For this review, take the finished solid that the model builds, in its own axes (mm). A direction names the side the tool comes from. Give positions to 0.01 mm unless a question says otherwise; leave off trailing zeros. Loops run counter-clockwise (first coordinate to the right, second up) from the corner with the lowest first, then second, coordinate; pieces in that order, holes last. Notation, with made-up numbers: (-1.75, 18) - (23.25, 18) arc R23 ccw to (23.25, 47) - close; hole circle Ø9 at (66, -6.75). An arc over 180 degrees is marked (long way). Put each result on its own line as item: value.
from build123d import *

# Parameters (mm, degrees)
CUT_EXTRUDE1_START = -1828.8
CUT_EXTRUDE1_DEPTH = 660.4
SKETCH3_R          = 2.38125
CUT_EXTRUDE3_DEPTH = 50.8
CUT_EXTRUDE4_REACH = 664.838
SKETCH4_R          = 2.413
CUT_EXTRUDE5_REACH = 664.838
SKETCH5_R          = 2.85115
SKETCH6_R          = 2.38125
CUT_EXTRUDE6_DEPTH = 663.837808315


with BuildPart() as part:
    # Cut-Extrude1: read off the stored shape, not the designer's step
    # Cut-Extrude1 outline → Cut-Extrude1 (new body)
    with BuildSketch(Plane.XY.offset(1828.8).offset(CUT_EXTRUDE1_START)):
        with BuildLine():
            Line((0, 50.546), (0, 0.254))
            ThreePointArc((0, 0.254), (0.074394878, 0.074394878), (0.254, 0))
            Line((0.254, 0), (25.146, 0))
            ThreePointArc((25.146, 0), (25.325605122, 0.074394878), (25.4, 0.254))
            Line((25.4, 0.254), (25.4, 50.546))
            ThreePointArc((25.4, 50.546), (25.325605122, 50.725605122), (25.146, 50.8))
            Line((25.146, 50.8), (0.254, 50.8))
            ThreePointArc((0.254, 50.8), (0.074394878, 50.725605122), (0, 50.546))
        make_face()
        with BuildLine():
            ThreePointArc((4.7625, 3.175), (3.639967985, 3.639967985), (3.175, 4.7625))
            Line((3.175, 4.7625), (3.175, 46.0375))
            ThreePointArc((3.175, 46.0375), (3.639967985, 47.160032015), (4.7625, 47.625))
            Line((4.7625, 47.625), (20.6375, 47.625))
            ThreePointArc((20.6375, 47.625), (21.760032015, 47.160032015), (22.225, 46.0375))
            Line((22.225, 46.0375), (22.225, 4.7625))
            ThreePointArc((22.225, 4.7625), (21.760032015, 3.639967985), (20.6375, 3.175))
            Line((20.6375, 3.175), (4.7625, 3.175))
        make_face(mode=Mode.SUBTRACT)
    extrude(amount=CUT_EXTRUDE1_DEPTH)

    # Sketch3 → Cut-Extrude3 (cut)
    with BuildSketch(Plane(origin=(0, 50.8, 0), x_dir=(1, 0, 0), z_dir=(0, 1, 0))):
        with Locations(Location((12.7, -25.4, 0), (0, 0, 270))):
            Circle(SKETCH3_R)
        with Locations(Location((12.7, -12.7, 0), (0, 0, 270))):
            Circle(SKETCH3_R)
        with Locations(Location((12.7, -38.1, 0), (0, 0, 270))):
            Circle(SKETCH3_R)
        with Locations(Location((12.7, -622.3, 0), (0, 0, 270))):
            Circle(SKETCH3_R)
        with Locations(Location((12.7, -635, 0), (0, 0, 270))):
            Circle(SKETCH3_R)
        with Locations(Location((12.7, -647.7, 0), (0, 0, 270))):
            Circle(SKETCH3_R)
    extrude(amount=-CUT_EXTRUDE3_DEPTH, mode=Mode.SUBTRACT)

    # Sketch4 → Cut-Extrude4 (cut, up to next)
    with BuildSketch(Plane(origin=(0, 50.8, 0), x_dir=(1, 0, 0), z_dir=(0, 1, 0)), mode=Mode.PRIVATE) as cut_extrude4_sk1:
        with Locations(Location((12.7, -532.289940881, 0), (0, 0, 270))):
            Circle(SKETCH4_R)
    cut_extrude4_tool1 = extrude(cut_extrude4_sk1.sketch, amount=-CUT_EXTRUDE4_REACH, mode=Mode.PRIVATE) & part.part
    # Sketch4 → Cut-Extrude4 (cut, up to next)
    with BuildSketch(Plane(origin=(0, 50.8, 0), x_dir=(1, 0, 0), z_dir=(0, 1, 0)), mode=Mode.PRIVATE) as cut_extrude4_sk2:
        with Locations(Location((12.7, -506.889940881, 0), (0, 0, 270))):
            Circle(SKETCH4_R)
    cut_extrude4_tool2 = extrude(cut_extrude4_sk2.sketch, amount=-CUT_EXTRUDE4_REACH, mode=Mode.PRIVATE) & part.part
    add(cut_extrude4_tool1.solids().sort_by_distance((12.7, 50.8, 532.289941))[0], mode=Mode.SUBTRACT)
    add(cut_extrude4_tool2.solids().sort_by_distance((12.7, 50.8, 506.889941))[0], mode=Mode.SUBTRACT)

    # Sketch5 → Cut-Extrude5 (cut, up to next)
    with BuildSketch(Plane(origin=(25.4, 0, 0), x_dir=(0, 0, -1), z_dir=(1, 0, 0)), mode=Mode.PRIVATE) as cut_extrude5_sk1:
        with Locations((-462.47685, 31.33725)):
            Circle(SKETCH5_R)
    cut_extrude5_tool1 = extrude(cut_extrude5_sk1.sketch, amount=-CUT_EXTRUDE5_REACH, mode=Mode.PRIVATE) & part.part
    # Sketch5 → Cut-Extrude5 (cut, up to next)
    with BuildSketch(Plane(origin=(25.4, 0, 0), x_dir=(0, 0, -1), z_dir=(1, 0, 0)), mode=Mode.PRIVATE) as cut_extrude5_sk2:
        with Locations((-429.82515, 31.33725)):
            Circle(SKETCH5_R)
    cut_extrude5_tool2 = extrude(cut_extrude5_sk2.sketch, amount=-CUT_EXTRUDE5_REACH, mode=Mode.PRIVATE) & part.part
    # Sketch5 → Cut-Extrude5 (cut, up to next)
    with BuildSketch(Plane(origin=(25.4, 0, 0), x_dir=(0, 0, -1), z_dir=(1, 0, 0)), mode=Mode.PRIVATE) as cut_extrude5_sk3:
        with Locations((-429.82515, 6.76275)):
            Circle(SKETCH5_R)
    cut_extrude5_tool3 = extrude(cut_extrude5_sk3.sketch, amount=-CUT_EXTRUDE5_REACH, mode=Mode.PRIVATE) & part.part
    # Sketch5 → Cut-Extrude5 (cut, up to next)
    with BuildSketch(Plane(origin=(25.4, 0, 0), x_dir=(0, 0, -1), z_dir=(1, 0, 0)), mode=Mode.PRIVATE) as cut_extrude5_sk4:
        with Locations((-462.47685, 6.76275)):
            Circle(SKETCH5_R)
    cut_extrude5_tool4 = extrude(cut_extrude5_sk4.sketch, amount=-CUT_EXTRUDE5_REACH, mode=Mode.PRIVATE) & part.part
    # Sketch5 → Cut-Extrude5 (cut, up to next)
    with BuildSketch(Plane(origin=(25.4, 0, 0), x_dir=(0, 0, -1), z_dir=(1, 0, 0)), mode=Mode.PRIVATE) as cut_extrude5_sk5:
        with Locations((-197.92315, 6.76275)):
            Circle(SKETCH5_R)
    cut_extrude5_tool5 = extrude(cut_extrude5_sk5.sketch, amount=-CUT_EXTRUDE5_REACH, mode=Mode.PRIVATE) & part.part
    # Sketch5 → Cut-Extrude5 (cut, up to next)
    with BuildSketch(Plane(origin=(25.4, 0, 0), x_dir=(0, 0, -1), z_dir=(1, 0, 0)), mode=Mode.PRIVATE) as cut_extrude5_sk6:
        with Locations((-230.57485, 31.33725)):
            Circle(SKETCH5_R)
    cut_extrude5_tool6 = extrude(cut_extrude5_sk6.sketch, amount=-CUT_EXTRUDE5_REACH, mode=Mode.PRIVATE) & part.part
    # Sketch5 → Cut-Extrude5 (cut, up to next)
    with BuildSketch(Plane(origin=(25.4, 0, 0), x_dir=(0, 0, -1), z_dir=(1, 0, 0)), mode=Mode.PRIVATE) as cut_extrude5_sk7:
        with Locations((-197.92315, 31.33725)):
            Circle(SKETCH5_R)
    cut_extrude5_tool7 = extrude(cut_extrude5_sk7.sketch, amount=-CUT_EXTRUDE5_REACH, mode=Mode.PRIVATE) & part.part
    # Sketch5 → Cut-Extrude5 (cut, up to next)
    with BuildSketch(Plane(origin=(25.4, 0, 0), x_dir=(0, 0, -1), z_dir=(1, 0, 0)), mode=Mode.PRIVATE) as cut_extrude5_sk8:
        with Locations((-230.57485, 6.76275)):
            Circle(SKETCH5_R)
    cut_extrude5_tool8 = extrude(cut_extrude5_sk8.sketch, amount=-CUT_EXTRUDE5_REACH, mode=Mode.PRIVATE) & part.part
    add(cut_extrude5_tool1.solids().sort_by_distance((25.4, 31.33725, 462.47685))[0], mode=Mode.SUBTRACT)
    add(cut_extrude5_tool2.solids().sort_by_distance((25.4, 31.33725, 429.82515))[0], mode=Mode.SUBTRACT)
    add(cut_extrude5_tool3.solids().sort_by_distance((25.4, 6.76275, 429.82515))[0], mode=Mode.SUBTRACT)
    add(cut_extrude5_tool4.solids().sort_by_distance((25.4, 6.76275, 462.47685))[0], mode=Mode.SUBTRACT)
    add(cut_extrude5_tool5.solids().sort_by_distance((25.4, 6.76275, 197.92315))[0], mode=Mode.SUBTRACT)
    add(cut_extrude5_tool6.solids().sort_by_distance((25.4, 31.33725, 230.57485))[0], mode=Mode.SUBTRACT)
    add(cut_extrude5_tool7.solids().sort_by_distance((25.4, 31.33725, 197.92315))[0], mode=Mode.SUBTRACT)
    add(cut_extrude5_tool8.solids().sort_by_distance((25.4, 6.76275, 230.57485))[0], mode=Mode.SUBTRACT)

    # Sketch6 → Cut-Extrude6 (cut, through all)
    with BuildSketch(Plane(origin=(25.4, 0, 0), x_dir=(0, 0, -1), z_dir=(1, 0, 0))):
        with Locations((-214.249, 40.48125)):
            Circle(SKETCH6_R)
        with Locations((-446.151, 40.48125)):
            Circle(SKETCH6_R)
    extrude(amount=-CUT_EXTRUDE6_DEPTH, mode=Mode.SUBTRACT)


solid = part.part
1) Insertion check: pin 1 Ø4 at (x, z) = (12.7, 12.7) entering from +Y; pin 2 Ø3.5 at (y, z) = (31.34, 197.92) entering from +X (3 decimals); pin 3 Ø5 at (y, z) = (6.76, 197.92) entering from +X. Each pin has a flat end and moves straight along its axis. Give the tip position at first contact, or say it passes through.
Geometry check:
pin 1: passes through
pin 2: stops at x = 3.175
pin 3: stops at x = 3.26
2) For faces 1 (the face through (3.175, 25, 326)), 2 (the face through (2, 24, 0)), list the 3-axis set-ups (+Z, -Z, +X, -X, +Y, -Y) from which the entire face can be reached by the end or side of a thin tool; tool diameter is ignored.
Geometry check:
face 1: +Z, -Z
face 2: -Z, +X, -X, +Y, -Y
3) Take a section at A-A on y = 17. State the section outline as (x, z) points (3 decimals).
Geometry check:
outline: (0, 0) - (3.175, 0) - (3.175, 660.4) - (0, 660.4) - close; (22.225, 0) - (25.4, 0) - (25.4, 660.4) - (22.225, 660.4) - close
4) Draft analysis for pull direction Y (two halves, no side actions). For faces 3 (the face through (25.4, 25, 326)), 4 (the face through (13, 0, 326)), 5 (the face through (13, 47.625, 326)), state which applies: pulls with the +Y half, pulls with the -Y half, needs draft (parallel to the pull), parting line crosses it, or undercut.
Geometry check:
face 3: needs draft
face 4: pulls with the -Y half
face 5: undercut
5) Wall thickness on line 1 (Z direction, x = 24.25, y = 31); line 2 (X direction, y = 21, z = 502) (3 decimals); line 3 (Y direction, x = 12.5, z = 375) (3 decimals): over which ranges is each line inside the solid? List them lowest first.
Geometry check:
line 1: z = 0 to 195.09, 200.75 to 227.74, 233.41 to 426.99, 432.66 to 459.65, 465.31 to 660.4
line 2: x = 0 to 3.175, 22.225 to 25.4
line 3: y = 0 to 3.175, 47.625 to 50.8
